Design review of the part built by this model. Coordinates are the model's own, in mm. A direction names the side the tool comes from. Round coordinates to 2 decimals unless told otherwise and drop trailing zeros. Loops run counter-clockwise (first coordinate to the right, second up) from the corner with the lowest first, then second, coordinate; pieces in that order, holes last. Notation, with made-up numbers: (-19.5, 86) - (28.5, 86) arc R25 cw to (28.5, 111) - close; hole circle Ø3 at (-25, 20.25). An arc over 180 degrees is marked (long way). Answer as CSV lines item,"result". Start each with the question number.
(1) Consider section C-C (x = 0). Count the separate pieces of the cut face and the enclosed holes in it, and give its area (3 significant figures).
(2) Consider section A-A (z = 8). Give the boundary of the cut face in (x, y), and give its area (3 significant figures).
(3) Consider section B-B (y = 0). Give the boundary of the cut face in (x, z).
(4) Wall thickness on L1, parallel to Z at x = -2.5, y = 0; L2, parallel to Y at x = -1.25, z = 3.5; L3, parallel to Y at x = 2.25, z = 14: over which ranges is each line inside the solid? List them lowest first.
(5) For faces 1 (the flat face through (0, -16.167, 24)), 2 (the flat face through (4.762, -17, 11)), 3 (the cylindrical face through (-0.07, 15.29, -12.36)), list the 3-axis set-ups (+Z, -Z, +X, -X, +Y, -Y) from which the entire face can be reached by the end or side of a thin tool; tool diameter is ignored.
(6) Mouldability with a two-part tool opening along X and no side actions: class faces 4 (the flat face through (0.07, -0.47, 25.9)), 5 (the cylindrical face through (0.61, -21.8, -3.02)), 6 (the flat face through (-4.762, -17, 11)), 7 (the cylindrical face through (0.09, 18.22, -14)) as released by +X, released by -X, zero draft, split by the parting line, or undercut.
(7) For P1, Ø3.5, axis at x = 0, z = 24.31, coming from the -Y side; P2, Ø2, axis at x = 1, y = 13, coming from the +Z side, all flat-tipped, find the tip position at first contact; note any pin that passes through.
from build123d import *

# Parameters (mm, degrees)
SKETCH1_R               = 2.2479
BOSS_EXTRUDE1_DEPTH     = 4.7625
SKETCH2_R               = 2.0193
CUT_EXTRUDE1_DEPTH      = 9.525
FILLET1_R               = 0.8255
FILLET2_R               = 5.08
FILLET3_R               = 5.08
CUT_EXTRUDE2_REACH      = 67.899
CUT_EXTRUDE2_END_RADIUS = 19.6596
SKETCH4_R               = 2.0193


with BuildPart() as part:
    # Sketch1 → Boss-Extrude1 (new, symmetric)
    with BuildSketch(Plane(origin=(0, 0, 0), x_dir=(0, 0, -1), z_dir=(1, 0, 0))):
        with BuildLine():
            Line((-31.1404, -25.6921), (22.8346, -25.6921))
            Line((22.8346, -25.6921), (22.8346, 3.821096341))
            Line((22.8346, 3.821096341), (22.8346, 13.103329243))
            ThreePointArc((22.8346, 13.103329243), (20.105248524, 16.996916667), (16.720065807, 20.336066331))
            Line((16.720065807, 20.336066331), (11.364530126, 23.747918844))
            ThreePointArc((11.364530126, 23.747918844), (5.82676412, 25.674209127), (0, 26.3271))
            Line((0, 26.3271), (-11.022257836, 20.35999918))
            ThreePointArc((-11.022257836, 20.35999918), (-16.769041287, 15.963050734), (-20.8778164, 10.006823511))
            Line((-20.8778164, 10.006823511), (-31.1404, -11.4046))
            Line((-31.1404, -11.4046), (-31.1404, -25.6921))
        make_face()
        with Locations(Location((13.3096, -20.9169, 0), (0, 0, 180))):
            Circle(SKETCH1_R, mode=Mode.SUBTRACT)
        with Locations(Location((-24.7904, -12.9921, 0), (0, 0, 180))):
            Circle(SKETCH1_R, mode=Mode.SUBTRACT)
        with BuildLine():
            Line((0, 19.6596), (0, 18.0721))
            ThreePointArc((0, 18.0721), (-9.710132252, -15.241854548), (16.378884958, 7.637599488))
            Line((16.378884958, 7.637599488), (17.81764857, 8.308505979))
            ThreePointArc((17.81764857, 8.308505979), (10.56309538, 16.580738468), (0, 19.6596))
        make_face(mode=Mode.SUBTRACT)
    extrude(amount=BOSS_EXTRUDE1_DEPTH, both=True)

    # Sketch2 → Cut-Extrude1 (cut)
    with BuildSketch(Plane.XZ.offset(25.6921)):
        with Locations(Location((0, -1.09474, 0), (0, 0, 270))):
            Circle(SKETCH2_R)
        with Locations(Location((0, 24.30526, 0), (0, 0, 270))):
            Circle(SKETCH2_R)
    extrude(amount=-CUT_EXTRUDE1_DEPTH, mode=Mode.SUBTRACT)

    # Fillet1
    fillet1_edges = [part.edges().sort_by_distance(p)[0] for p in [
        (0, -25.6921, -22.8346),
        (0, -25.6921, 31.1404),
        (0, -11.4046, 31.1404),
    ]]
    fillet(fillet1_edges, radius=FILLET1_R)

    # Chamfer1
    # the kernel refuses this chamfer: 3.302, 1.906410589 mm, written as the material it takes off along each edge
    with BuildSketch(Plane(origin=(-12.550145682, 7.637599488, -16.378884958), x_dir=(0, -0.9448116509539838, -0.32761401713236815), z_dir=(1, 0, 0))) as chamfer1_piece_1_section:
        with BuildLine():
            Line((3.115058273, 0), (-0.285434968, 1.681623622))
            Line((-0.285434968, 1.681623622), (-0.351127983, 1.674862743))
            ThreePointArc((-0.351127983, 1.674862743), (-0.152815077, 0.839772605), (-0.065693014, -0.00676088))
            Line((-0.065693014, -0.00676088), (0.00676088, -0.065693014))
            ThreePointArc((0.00676088, -0.065693014), (1.557097323, 0.026529257), (3.110868588, -0.065906966))
            Line((3.110868588, -0.065906966), (3.115058273, 0))
        make_face()
    chamfer1_piece_1 = extrude(amount=25.100291364, mode=Mode.PRIVATE)
    chamfer1_piece_1 = chamfer1_piece_1 & Plane(origin=(0, 0, 0), x_dir=(0, 0.4226182617407049, -0.9063077870366475), z_dir=(1, 0, 0)) * Cylinder(19.6596, 63, mode=Mode.PRIVATE)
    add(chamfer1_piece_1, mode=Mode.SUBTRACT)
    with BuildSketch(Plane(origin=(12.550145682, 18.0721, 0), x_dir=(0, -0.10237552272911479, 0.9947458229849173), z_dir=(-1, 0, 0))) as chamfer1_piece_2_section:
        with BuildLine():
            Line((3.115058273, 0), (-0.285434968, 1.681623622))
            Line((-0.285434968, 1.681623622), (-0.351127983, 1.674862743))
            ThreePointArc((-0.351127983, 1.674862743), (-0.152815077, 0.839772605), (-0.065693014, -0.00676088))
            Line((-0.065693014, -0.00676088), (0.00676088, -0.065693014))
            ThreePointArc((0.00676088, -0.065693014), (1.557097323, 0.026529257), (3.110868588, -0.065906966))
            Line((3.110868588, -0.065906966), (3.115058273, 0))
        make_face()
    chamfer1_piece_2 = extrude(amount=25.100291364, mode=Mode.PRIVATE)
    chamfer1_piece_2 = chamfer1_piece_2 & Plane(origin=(0, 0, 0), x_dir=(0, 0.4226182617407049, -0.9063077870366475), z_dir=(1, 0, 0)) * Cylinder(19.6596, 63, mode=Mode.PRIVATE)
    add(chamfer1_piece_2, mode=Mode.SUBTRACT)

    # Fillet2
    fillet2_edges = [part.edges().sort_by_distance(p)[0] for p in [
        (0, 26.3271, 0),
        (0, 23.747918844, -11.364530126),
        (0, 20.336066331, -16.720065807),
        (0, 13.103329243, -22.8346),
    ]]
    fillet(fillet2_edges, radius=FILLET2_R)

    # Fillet3
    fillet3_edges = [part.edges().sort_by_distance(p)[0] for p in [
        (0, 17.823556008, 2.98691306),
        (0, 4.825497693, -17.415951608),
        (0, 8.2447084, -17.847259049),
        (0, 19.659474186, 0.070334171),
    ]]
    fillet(fillet3_edges, radius=FILLET3_R)

    # Cut-Extrude2: up to this cylinder (the profile starts outside it)
    cut_extrude2_end = Plane(origin=(0, 0, 0), z_dir=(-1, 0, 0)) * Cylinder(CUT_EXTRUDE2_END_RADIUS, 176.1172, mode=Mode.PRIVATE)
    # Sketch4 → Cut-Extrude2 (cut, up to the surface)
    with BuildSketch(Plane(origin=(0, 22.041992588, -14.042297966), x_dir=(1, 0, 0), z_dir=(0, 0.8433914458128872, -0.5372996083468217)), mode=Mode.PRIVATE) as cut_extrude2_sk1:
        with Locations(Location((0, 0, 0), (0, 0, 270))):
            Circle(SKETCH4_R)
    cut_extrude2_tool1 = extrude(cut_extrude2_sk1.sketch, amount=-CUT_EXTRUDE2_REACH, mode=Mode.PRIVATE) - cut_extrude2_end
    add(cut_extrude2_tool1.solids().sort_by_distance((0, 22.041993, -14.042298))[0], mode=Mode.SUBTRACT)


solid = part.part
Determined:
1,separate pieces,"2"
1,enclosed holes,"2"
1,area,"1,120 mm^2"
2,outline,"(-4.76, -25.69) - (4.76, -25.69) - (4.76, -16.2) - (-4.76, -16.2) - close; (-4.76, 16.2) - (4.76, 16.2) - (4.76, 22) - (-4.76, 22) - close"
2,area,"146 mm^2"
3,outline,"(-4.76, -22.83) - (4.76, -22.83) - (4.76, -18.07) - (-4.76, -18.07) - close; (-4.76, 18.07) - (4.76, 18.07) - (4.76, 25.67) - (-4.76, 25.67) - close"
4,L1,"z = -22.83 to -18.07, 18.07 to 25.67"
4,L2,"y = -25.69 to -17.73, 17.74 to 24.43"
4,L3,"y = -25.69 to -11.43, 11.43 to 18.44"
5,face 1,"-Y"
5,face 2,"+Z, -Z, +X, +Y, -Y"
5,face 3,"+X, -X"
6,face 4,"zero draft"
6,face 5,"undercut"
6,face 6,"released by -X"
6,face 7,"undercut"
7,P1,"stops at y = -16.17"
7,P2,"stops at z = 19.8"
